Autodesk Inventor part; units mm, degrees
ref_plane "YZ Plane" through (0, 0, 0) normal (1, 0, 0) x (0, 1, 0)
ref_plane "XZ Plane" through (0, 0, 0) normal (0, 1, 0) x (-1, 0, 0)
ref_plane "XY Plane" through (0, 0, 0) normal (0, 0, 1) x (1, 0, 0)
sketch "Sketch1" plane through (0, 0, 0) normal (0, 1, 0) x (-1, 0, 0)
  line L0 (0, 0) -> (6, 0)
  line L1 (6, 0) -> (6, -23)
  line L2 (6, -23) -> (0, -23)
  line L3 (0, -23) -> (0, 0)
  circle A0 centre (3, -2.5) radius 1.5
  circle A1 centre (3, -20.5) radius 1.75
  dimension "d0" = 6
  dimension "d1" = 23
  dimension "d2" = 6
  dimension "d4" = 3
  dimension "d5" = 3.5
  dimension "d6" = 2.5
  dimension "d7" = 2.5
extrude "Extrusion1" add sketch "Sketch1" along normal blind 3
fillet "Fillet1" radius 3 1 edges at (-6, 1.5, 0)
fillet "Fillet2" radius 3 3 edges at (0, 1.5, 0) (-6, 1.5, -23) (0, 1.5, -23)
properties part number "reverse gear drag link"
The listing builds one solid part. Answer for the finished solid, in the listing's coordinates (mm). Coordinates: 2 decimals unless noted, no trailing zeros. Loops run counter-clockwise (first coordinate to the right, second up) from the corner with the lowest first, then second, coordinate; pieces in that order, holes last. Notation, with made-up numbers: (86.5, 23.25) -> (127.5, 23.25) arc R12 cw to (127.5, 30.25) -> close; hole circle Ø10 at (-22.5, 39). An arc over 180 degrees is marked (long way). Answer in a Markdown table with one row per item. Add a question column.
1. The part is cut by section C-C, the plane x = -3.7. Write down the section's boundary in (y, z).
2. The part is cut by section B-B, the plane z = -3.75. Write down the section's boundary in (x, y).
3. The part is cut by section A-A, the plane y = 0.5. Count the separate pieces of the cut face and the enclosed holes in it, then the cut area to 3 significant figures.
4. The part is cut by section D-D, the plane z = -21.25. Write down the section's boundary in (x, y).
5. Determine the mould class of faces 1 (the flat face through (-3, 0, -11)), 2 (the cylindrical face through (-0.9, 1.52, -0.86)), 3 (the cylindrical face through (-2.772, 1.479, -22.235)), 4 (the cylindrical face through (-3.69, 1.48, -1.17)) for opening direction X: +X half, -X half, draft (parallel to the pull), parting line (faces both ways), or undercut.
6. Consider line 1 (Z direction, x = -3, y = 1.4); line 2 (Z direction, x = -2.4, y = 1.15); line 3 (Z direction, x = -5.3, y = 1.85). Determine where each line is inside the solid, lowest interval first. Write a range as [from, to].
7. Flat-ended cylindrical pins translate along their axes: P1, Ø3, axis at x = -3, z = -20.5, coming from the +Y side; P2, Ø1, axis at x = -4, y = 0.5, coming from the +Z side. Find the tip coordinate at first contact, or state that the pin passes through.
Answer below:
| question | item | result |
|---|---|---|
| 1 | outline | (0, -22.92) -> (3, -22.92) -> (3, -22.1) -> (0, -22.1) -> close; (0, -18.9) -> (3, -18.9) -> (3, -3.83) -> (0, -3.83) -> close; (0, -1.17) -> (3, -1.17) -> (3, -0.08) -> (0, -0.08) -> close |
| 2 | outline | (-6, 0) -> (-3.83, 0) -> (-3.83, 3) -> (-6, 3) -> close; (-2.17, 0) -> (0, 0) -> (0, 3) -> (-2.17, 3) -> close |
| 3 | separate pieces | 1 |
| 3 | enclosed holes | 2 |
| 3 | area | 114 mm2 |
| 4 | outline | (-5.73, 0) -> (-4.58, 0) -> (-4.58, 3) -> (-5.73, 3) -> close; (-1.42, 0) -> (-0.27, 0) -> (-0.27, 3) -> (-1.42, 3) -> close |
| 5 | face 1 | draft |
| 5 | face 2 | +X half |
| 5 | face 3 | undercut |
| 5 | face 4 | undercut |
| 6 | line 1 | [-23, -22.25], [-18.75, -4], [-1, 0] |
| 6 | line 2 | [-22.94, -22.14], [-18.86, -3.87], [-1.13, -0.06] |
| 6 | line 3 | [-21.93, -1.07] |
| 7 | P1 | through |
| 7 | P2 | z = -0.04 |
